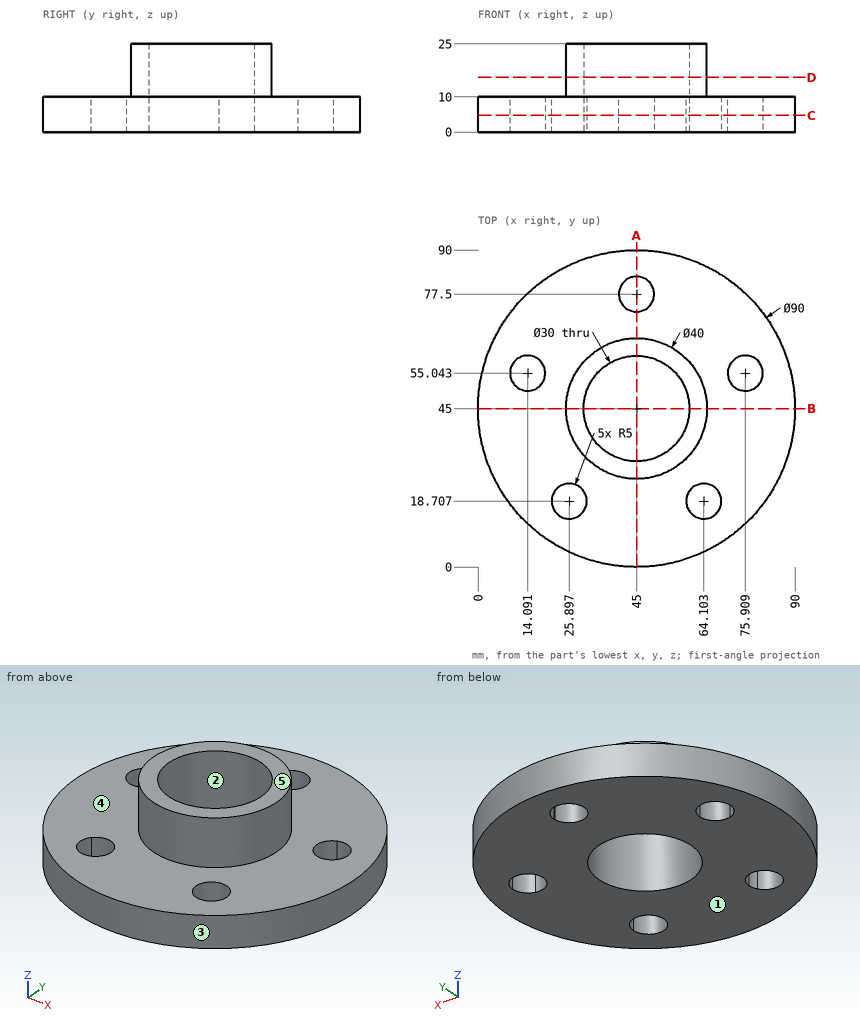
Verification items for this drawing (mm, ordinates from the low corner). A direction names the side the tool comes from. Give positions to 0.01 mm unless a question says otherwise; leave off trailing zeros. Loops run counter-clockwise (first coordinate to the right, second up) from the corner with the lowest first, then second, coordinate; pieces in that order, holes last. Notation, with made-up numbers: M -25.75,29.25 L -2.75,29.25 A6 ccw -2.75,35.25 Z; hole C 79,24 d8. An arc over 180 degrees is marked long. Return JSON: item names as keys, results as strings. Group by question number.
1. Cross-section at A-A on x = 45. Record the boundary of the cut face in (y, z).
2. Cross-section at C-C on z = 4.75. Record the boundary of the cut face in (x, y) (1 decimal), plus the area to 3 significant figures.
3. Mould release check, pull along X, two halves, no side actions. Record for the marked faces 1, 2 and 3: released by +X, released by -X, zero draft, split by the parting line, or undercut.
4. Thickness scan on L1, parallel to Y at x = 45, z = 7.75; L2, parallel to Y at x = 45, z = 14.25. Record the ranges inside material, lowest first.
5. Go/stop test with flat-tipped pins: pin 1 (6 mm diameter, centred on x = 25, z = 5.5, fed in from +Y) (1 decimal); pin 2 (4 mm diameter, centred on y = 56, z = 20, fed in from -X); pin 3 (8 mm diameter, centred on x = 55.5, y = 77.5, fed in from +Z). Record where each tip stops, or that it passes through.
6. Tool access check on the marked faces 4 and 5. Record the directions out of +Z, -Z, +X, -X, +Y, -Y that give a thin tool (end or side, any length) a straight path to the whole face; none if there is none.
7. Cross-section at D-D on z = 15.5. Record the boundary of the cut face in (x, y), plus the area to 3 significant figures.
8. Cross-section at B-B on y = 45. Record the boundary of the cut face in (x, z).
Return value:
{
 "1": {"outline": "M 0,0 L 30,0 L 30,25 L 25,25 L 25,10 L 0,10 Z; M 60,0 L 72.5,0 L 72.5,10 L 65,10 L 65,25 L 60,25 Z; M 82.5,0 L 90,0 L 90,10 L 82.5,10 Z"},
 "2": {"outline": "C 45,45 d90; hole C 14.1,55 d10; hole C 25.9,18.7 d10; hole C 45,45 d30; hole C 45,77.5 d10; hole C 64.1,18.7 d10; hole C 75.9,55 d10", "area": "5,260 mm^2"},
 "3": {"face 1": "zero draft", "face 2": "undercut", "face 3": "split by the parting line"},
 "4": {"L1": "0 to 30, 60 to 72.5, 82.5 to 90", "L2": "25 to 30, 60 to 65"},
 "5": {"pin 1": "y = 86.7", "pin 2": "x = 27.14", "pin 3": "z = 10"},
 "6": {"face 4": "+Z", "face 5": "+Z, +X, -X, +Y, -Y"},
 "7": {"outline": "C 45,45 d40; hole C 45,45 d30", "area": "550 mm^2"},
 "8": {"outline": "M 0,0 L 30,0 L 30,25 L 25,25 L 25,10 L 0,10 Z; M 60,0 L 90,0 L 90,10 L 65,10 L 65,25 L 60,25 Z"}
}
